Print and shaded views of the part. All mm, measured from the part's lowest x, y and z. Round coordinates to 2 decimals unless told otherwise and drop trailing zeros. Loops run counter-clockwise (first coordinate to the right, second up) from the corner with the lowest first, then second, coordinate; pieces in that order, holes last. Notation, with made-up numbers: (56.25, -1) - (66.25, -1) arc R31 ccw to (66.25, 31) - close; hole circle Ø10 at (53, 45.5). An arc over 180 degrees is marked (long way). Use one line per item in the form item = value.
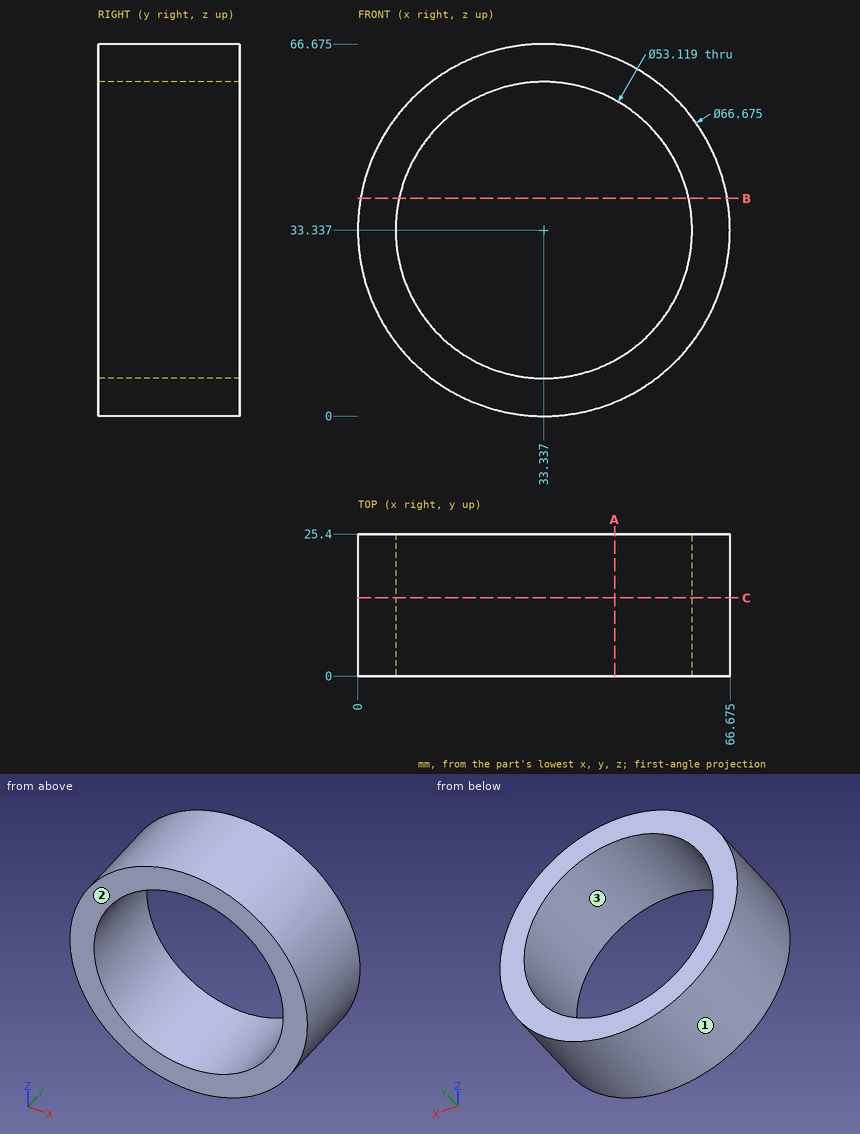
1) Slice it at A-A (x = 46). Write the cut outline in (y, z) (1 decimal).
Report:
outline = (0, 2.5) - (25.4, 2.5) - (25.4, 10) - (0, 10) - close; (0, 56.7) - (25.4, 56.7) - (25.4, 64.2) - (0, 64.2) - close
2) Drill centre lines: probe 1 along X at (y, z) = (21.25, 33.5) (1 decimal); probe 2 along X at (y, z) = (12.25, 49.5) (1 decimal); probe 3 along Z at (x, y) = (16, 6.75) (1 decimal). Where is each one in solid material? Low to high.
Report:
probe_1 = 0 to 6.8, 59.9 to 66.7
probe_2 = 4.2 to 12.3, 54.4 to 62.5
probe_3 = 4.9 to 13.2, 53.5 to 61.8
3) Slice it at C-C (y = 14). Write the cut outline in (x, z) (1 decimal).
Report:
outline = circle Ø66.7 at (33.3, 33.3); hole circle Ø53.1 at (33.3, 33.3)
4) Flat gauge pins, fed straight in: pin 1 (1.5 mm diameter, centred on y = 13.5, z = 12.5, fed in from -X); pin 2 (4 mm diameter, centred on x = 35.5, y = 15, fed in from -Z); pin 3 (1.5 mm diameter, centred on y = 3, z = 53.5, fed in from -X) (1 decimal). Where does each tip first touch, or does it go through?
Report:
pin_1 = 6.73
pin_2 = 0
pin_3 = 6.2
5) Slice it at B-B (z = 39). Write the cut outline in (x, y) (1 decimal).
Report:
outline = (0.5, 0) - (7.4, 0) - (7.4, 25.4) - (0.5, 25.4) - close; (59.3, 0) - (66.2, 0) - (66.2, 25.4) - (59.3, 25.4) - close
6) Two-plate mould, pull along Z, no slides. Class the marked faces 1, 2 and 3: +Z half, -Z half, draft (parallel to the pull), parting line (faces both ways), or undercut.
Report:
face_1 = parting line
face_2 = draft
face_3 = undercut
